from build123d import *

# Parameters (mm, degrees)
SKETCH1_R               = 101.6
SKETCH1_R_2             = 99.06
BOSS_EXTRUDE1_DEPTH     = 165.1
CUT_EXTRUDE1_DEPTH      = 165.1
FILLET1_R               = 12.7
SKETCH3_R               = 1.397
CUT_EXTRUDE2_DEPTH      = 219.867837001
CUT_EXTRUDE2_DEPTH_BACK = 219.867837001
SKETCH4_R               = 9.525
CUT_EXTRUDE3_DEPTH      = 219.867837003


with BuildPart() as part:
    # Sketch1 → Boss-Extrude1 (new body)
    with BuildSketch(Plane(origin=(0, 0, 0), x_dir=(1, 0, 0), z_dir=(0, 1, 0))):
        with Locations(Location((0, 0, 0), (0, 0, 270))):
            Circle(SKETCH1_R)
        with Locations(Location((0, 0, 0), (0, 0, 270))):
            Circle(SKETCH1_R_2, mode=Mode.SUBTRACT)
    extrude(amount=BOSS_EXTRUDE1_DEPTH)

    # Sketch2 → Cut-Extrude1 (cut)
    with BuildSketch(Plane(origin=(0, 0, 0), x_dir=(1, 0, 0), z_dir=(0, 1, 0))):
        Polygon((571.962381958, -80.384070579), (100.611235784, -14.139987058), (0, 0), (-100.611235784, -14.139987058), (-571.962381958, -80.384070579), (-571.962381958, -1032.350838067), (571.962381958, -1032.350838067), align=None)
    extrude(amount=CUT_EXTRUDE1_DEPTH, mode=Mode.SUBTRACT)

    # Fillet1
    fillet1_edges = [part.edges().sort_by_distance(p)[0] for p in [
        (-99.353595337, 0, 13.963237219),
        (99.353595337, 165.1, 13.963237219),
        (-99.353595337, 165.1, 13.963237219),
        (99.353595337, 0, 13.963237219),
    ]]
    fillet(fillet1_edges, radius=FILLET1_R)

    # Sketch3 → Cut-Extrude2 (cut, two sides)
    with BuildSketch(Plane(origin=(0, 0, 0), x_dir=(0, 0, -1), z_dir=(1, 0, 0))) as cut_extrude2_sk:
        with Locations((0.084012942, 29.1846)):
            Circle(SKETCH3_R)
        with Locations((0.022897636, 129.159100035)):
            Circle(SKETCH3_R)
    extrude(amount=CUT_EXTRUDE2_DEPTH, mode=Mode.SUBTRACT)
    extrude(cut_extrude2_sk.sketch, amount=-CUT_EXTRUDE2_DEPTH_BACK, mode=Mode.SUBTRACT)

    # Sketch4 → Cut-Extrude3 (cut, through all)
    with BuildSketch(Plane.XY):
        with Locations((0, 20.32)):
            Circle(SKETCH4_R)
    extrude(amount=-CUT_EXTRUDE3_DEPTH, mode=Mode.SUBTRACT)


solid = part.part
Could you check a few things on this model? Use its own coordinates, in mm. A direction names the side the tool comes from. Give positions to 0.01 mm unless a question says otherwise; leave off trailing zeros. Write each loop counter-clockwise with the first axis right and the second up, starting at its lowest first coordinate (ties: lowest second). Pieces come first, ordered by that corner, then holes. Notation, with made-up numbers: (15, 15) -> (26, 15) arc R14 cw to (26, 35) -> close; hole circle Ø11 at (83, 38.5). An arc over 180 degrees is marked (long way). Write each question's results on one line, items separated by ' | '. Start each with the question number.
Q1. I need wall thicknesses on probe 1 along X at (y, z) = (116, 0); probe 2 along Z at (x, y) = (0, 125); probe 3 along X at (y, z) = (11, -5.5). Which ranges of each line are inside material? Lowest first, please.
Q2. Which directions (+Z, -Z, +X, -X, +Y, -Y) give clear straight access to the entire face, cutting with the end or side of a thin tool? Please do faces 4 (the face through (-99.87, 3.62, 10.18)), 5 (the face through (2.37, 81.39, -99.03)), 6 (the face through (-99.846, 161.281, 10.375)).
Q3. We'd pull the mould along Y, two halves only. Please class faces 1 (the face through (99.83, 161.48, 10.17)), 2 (the face through (8.8, 16.67, -100.08)), 3 (the face through (99.83, 3.62, 10.17)): +Y half, -Y half, draft (parallel to the pull), parting line (faces both ways), or undercut.
Q4. Suppose I cut it at B-B, the plane y = 20.32. List the corners of the cut face in (x, z) for me (3 decimals).
Q5. Suppose I cut it at A-A, the plane x = 0. List the corners of the cut face in (y, z) for me (3 decimals).
Q6. Suppose I cut it at C-C, the plane y = 62.5. List the corners of the cut face in (x, z) for me, and give its area (3 significant figures).
Q7. I'm going to push flat-ended pins straight in: pin 1 Ø17 at (x, y) = (0, 20.32) entering from +Z; pin 2 Ø1.5 at (x, y) = (-53, 55.5) entering from +Z; pin 3 Ø12 at (x, y) = (39.5, 91.5) entering from +Z; pin 4 Ø1 at (x, y) = (40, 38) entering from -Z. Where does each tip first touch, or does it pass through?
Outcome:
1) probe 1: -101.6 to -99.06, 99.06 to 101.6 | probe 2: -101.6 to -99.06 | probe 3: -101.45 to -98.91, 98.91 to 101.45
2) face 4: +Z, -Y | face 5: +Y, -Y | face 6: +Z, +Y
3) face 1: +Y half | face 2: undercut | face 3: -Y half
4) outline: (-100.611, 14.14) arc R101.6 ccw to (-9.525, -101.153) -> (-9.525, -98.601) arc R99.06 cw to (-98.096, 13.786) -> close; (9.525, -101.153) arc R101.6 ccw to (100.611, 14.14) -> (98.096, 13.786) arc R99.06 cw to (9.525, -98.601) -> close
5) outline: (0, -101.6) -> (10.795, -101.6) -> (10.795, -99.06) -> (0, -99.06) -> close; (29.845, -101.6) -> (165.1, -101.6) -> (165.1, -99.06) -> (29.845, -99.06) -> close
6) outline: (-100.61, 14.14) arc R101.6 ccw (long way) to (100.61, 14.14) -> (98.1, 13.79) arc R99.06 cw (long way) to (-98.1, 13.79) -> close | area: 872 mm2
7) pin 1: through | pin 2: z = -83.21 | pin 3: z = -87.99 | pin 4: z = -93.61
